Check sheet for the drawn part. Datum: minimum x, y, z corner. Units: mm. A direction names the side the tool comes from. Give positions to 0.01 mm unless a question says otherwise; leave off trailing zeros. Order: outer loops, then holes, each group sorted by start corner. A loop starts at its lowest first (then second) coordinate and runs counter-clockwise, first axis right, second up. Notation, with made-up numbers: M 1.5,55 L 32.5,55 A14 cw 32.5,62 Z; hole C -18.75,-20 d1. An arc over 180 degrees is marked long. Put each result on its own line as item: value. Start each with the question number.
Q1. Section check A-A on x = 6.35. State how many separate pieces and enclosed holes the cut face has.
Q2. Section check B-B on z = 10.16. Record the cut outline in (x, y) (1 decimal).
Q3. Access from +Z, -Z, +X, -X, +Y, -Y to the whole of each face (thin tool, end or side, straight path). Record for the marked faces 1 and 2.
Q4. Section check C-C on z = 5. Record the cut outline in (x, y) (1 decimal).
Q5. Mould release check, pull along Z, two halves, no side actions. Record for the marked faces 3, 4 and 5: +Z half, -Z half, draft (parallel to the pull), parting line (faces both ways), or undercut.
Q6. Material ranges on L1, parallel to X at y = 0.85, z = 6.35; L2, parallel to X at y = 1.75, z = 5.75 (1 decimal); L3, parallel to Y at x = 6.25, z = 12, recorded low to high.
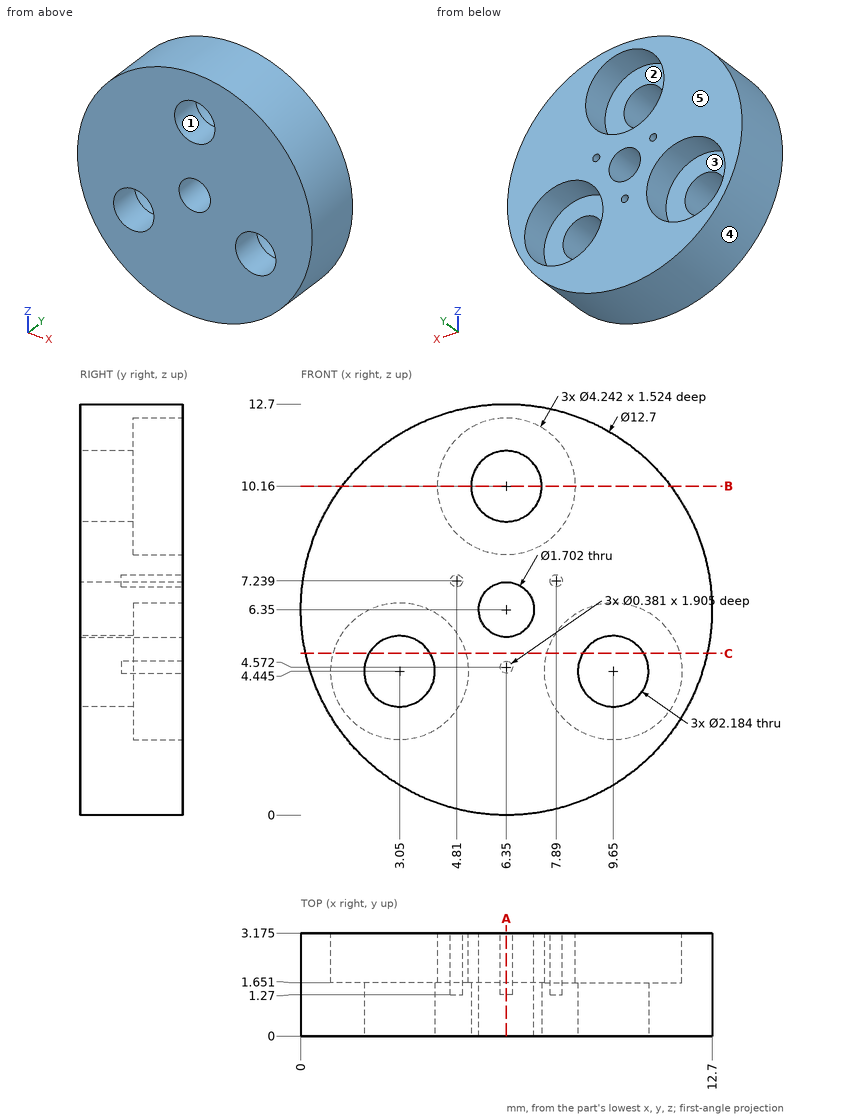
Results found:
1. separate pieces: 3
1. enclosed holes: 0
2. outline: M 1.3,0 L 5.3,0 L 5.3,1.7 L 4.2,1.7 L 4.2,3.2 L 1.3,3.2 Z; M 7.4,0 L 11.4,0 L 11.4,3.2 L 8.5,3.2 L 8.5,1.7 L 7.4,1.7 Z
3. face 1: +Y, -Y
3. face 2: +Y
4. outline: M 0.1,0 L 2.1,0 L 2.1,1.7 L 1,1.7 L 1,3.2 L 0.1,3.2 Z; M 4,0 L 8.7,0 L 8.7,1.7 L 7.6,1.7 L 7.6,3.2 L 5.1,3.2 L 5.1,1.7 L 4,1.7 Z; M 10.6,0 L 12.6,0 L 12.6,3.2 L 11.7,3.2 L 11.7,1.7 L 10.6,1.7 Z
5. face 3: undercut
5. face 4: parting line
5. face 5: draft
6. L1: x = 0 to 5.5, 7.2 to 12.7
6. L2: x = 0 to 1.4, 4.7 to 5.7, 7 to 8, 11.3 to 12.7
6. L3: y = 0 to 1.65
